Could you check a few things on this model? Use its own coordinates, in mm. Face numbers are marked on the shaded views. A direction names the side the tool comes from. Give positions to 0.01 mm unless a question says otherwise; leave off trailing zeros. Loops run counter-clockwise (first coordinate to the right, second up) from the corner with the lowest first, then second, coordinate; pieces in that order, holes last. Notation, with made-up numbers: (-3.75, 20.25) -> (28.25, 20.25) arc R21 cw to (28.25, 49.25) -> close; hole circle Ø9 at (73, 59). An arc over 180 degrees is marked (long way). Put each result on its own line as item: value.
```python
from build123d import *

# Parameters (mm, degrees)
BOSS_EXTRUDE1_DEPTH = 25.4
SKETCH3_R           = 2.159
CUT_EXTRUDE3_DEPTH  = 49.912809743
CUT_EXTRUDE4_DEPTH  = 49.050496574
CHAMFER1_SIZE       = 3.175


with BuildPart() as part:
    # Sketch2 → Boss-Extrude1 (new, symmetric)
    with BuildSketch(Plane.XY):
        Polygon((-14.859, 0), (-14.225031823, 0), (14.859, 0), (14.859, -26.67), (30.861, -26.67), (30.861, -28.194), (13.335, -28.194), (13.335, -1.524), (-13.335, -1.524), (-13.335, -28.194), (-30.861, -28.194), (-30.861, -26.67), (-14.859, -26.67), align=None)
    extrude(amount=BOSS_EXTRUDE1_DEPTH, both=True)

    # Sketch3 → Cut-Extrude3 (cut, through all)
    with BuildSketch(Plane(origin=(0, 0, 0), x_dir=(1, 0, 0), z_dir=(0, 1, 0))):
        with Locations(Location((0, -15.875, 0), (0, 0, 270))):
            Circle(SKETCH3_R)
        with Locations(Location((0, 15.875, 0), (0, 0, 270))):
            Circle(SKETCH3_R)
        with Locations(Location((0, 0, 0), (0, 0, 270))):
            Circle(SKETCH3_R)
    extrude(amount=-CUT_EXTRUDE3_DEPTH, mode=Mode.SUBTRACT)

    # Sketch9 → Cut-Extrude4 (cut, through all)
    with BuildSketch(Plane(origin=(0, -26.67, 0), x_dir=(1, 0, 0), z_dir=(0, 1, 0))):
        with BuildLine():
            Line((26.4668, 19.0373), (26.4668, 12.7127))
            ThreePointArc((26.4668, 12.7127), (22.8981, 9.144), (19.3294, 12.7127))
            Line((19.3294, 12.7127), (19.3294, 19.0373))
            ThreePointArc((19.3294, 19.0373), (22.8981, 22.606), (26.4668, 19.0373))
        make_face()
        with BuildLine():
            Line((-26.4668, 19.0373), (-26.4668, 12.7127))
            ThreePointArc((-26.4668, 12.7127), (-22.8981, 9.144), (-19.3294, 12.7127))
            Line((-19.3294, 12.7127), (-19.3294, 19.0373))
            ThreePointArc((-19.3294, 19.0373), (-22.8981, 22.606), (-26.4668, 19.0373))
        make_face()
        with BuildLine():
            Line((26.4668, -19.0373), (26.4668, -12.7127))
            ThreePointArc((26.4668, -12.7127), (22.8981, -9.144), (19.3294, -12.7127))
            Line((19.3294, -12.7127), (19.3294, -19.0373))
            ThreePointArc((19.3294, -19.0373), (22.8981, -22.606), (26.4668, -19.0373))
        make_face()
        with BuildLine():
            Line((-26.4668, -19.0373), (-26.4668, -12.7127))
            ThreePointArc((-26.4668, -12.7127), (-22.8981, -9.144), (-19.3294, -12.7127))
            Line((-19.3294, -12.7127), (-19.3294, -19.0373))
            ThreePointArc((-19.3294, -19.0373), (-22.8981, -22.606), (-26.4668, -19.0373))
        make_face()
    extrude(amount=-CUT_EXTRUDE4_DEPTH, mode=Mode.SUBTRACT)

    # Chamfer1
    chamfer1_edges = [part.edges().sort_by_distance(p)[0] for p in [
        (-30.861, -27.432, 25.4),
        (30.861, -27.432, -25.4),
        (-30.861, -27.432, -25.4),
        (30.861, -27.432, 25.4),
    ]]
    chamfer(chamfer1_edges, length=CHAMFER1_SIZE)


solid = part.part
```
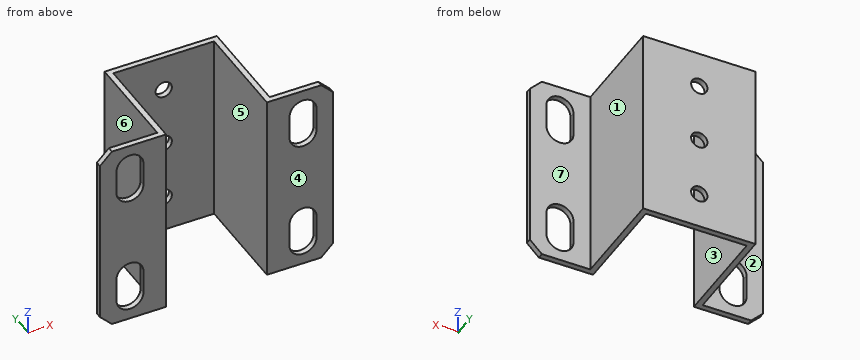
1. Thinking about a two-plate mould opening in X: for the marked faces 1, 2 and 3, which applies, pulls with the +X half, pulls with the -X half, needs draft (parallel to the pull), parting line crosses it, or undercut?
Recorded:
face 1: pulls with the +X half
face 2: needs draft
face 3: undercut
2. If we section it at A-A (y = -21.75): List the corners of the cut face in (x, z) for me (3 decimals), then the cut area to 3 significant figures.
Recorded:
outline: (-14.859, -25.4) -> (-13.335, -25.4) -> (-13.335, 25.4) -> (-14.859, 25.4) -> close; (13.335, -25.4) -> (14.859, -25.4) -> (14.859, 25.4) -> (13.335, 25.4) -> close
area: 155 mm^2
3. If we section it at B-B (x = 0): List the corners of the cut face in (y, z) for me, then the cut area to 3 significant figures.
Recorded:
outline: (-1.52, -25.4) -> (0, -25.4) -> (0, -18.03) -> (-1.52, -18.03) -> close; (-1.52, -13.72) -> (0, -13.72) -> (0, -2.16) -> (-1.52, -2.16) -> close; (-1.52, 2.16) -> (0, 2.16) -> (0, 13.72) -> (-1.52, 13.72) -> close; (-1.52, 18.03) -> (0, 18.03) -> (0, 25.4) -> (-1.52, 25.4) -> close
area: 57.7 mm^2
4. For the marked faces 4, 5, 6 and 7, which set-ups out of +Z, -Z, +X, -X, +Y, -Y let a thin tool reach every point of the face, with its end or its side?
Recorded:
face 4: +Z, -Z, +X, -X, -Y
face 5: +Z, -Z, -Y
face 6: +Z, -Z, -X, +Y
face 7: +Z, -Z, +X, +Y
5. I'm going to push flat-ended pins straight in: pin 1 (8 mm diameter, centred on y = -15, z = -5.5, fed in from +X); pin 2 (8 mm diameter, centred on x = 24.5, z = -2.5, fed in from +Y); pin 3 (3 mm diameter, centred on y = -21.5, z = -15, fed in from -X). Where does each tip first touch, or does it pass through?
Recorded:
pin 1: stops at x = 14.86
pin 2: stops at y = -26.67
pin 3: stops at x = -14.86
6. If we section it at D-D (z = -5.5): List the corners of the cut face in (x, y) for me (3 decimals), then the cut area to 3 significant figures.
Recorded:
outline: (-30.861, -28.194) -> (-13.335, -28.194) -> (-13.335, -1.524) -> (13.335, -1.524) -> (13.335, -28.194) -> (30.861, -28.194) -> (30.861, -26.67) -> (14.859, -26.67) -> (14.859, 0) -> (-14.859, 0) -> (-14.859, -26.67) -> (-30.861, -26.67) -> close
area: 175 mm^2
7. If we section it at C-C (z = 0): List the corners of the cut face in (x, y) for me (3 decimals), then the cut area to 3 significant figures.
Recorded:
outline: (-30.861, -28.194) -> (-13.335, -28.194) -> (-13.335, -1.524) -> (-2.159, -1.524) -> (-2.159, 0) -> (-14.859, 0) -> (-14.859, -26.67) -> (-30.861, -26.67) -> close; (2.159, -1.524) -> (13.335, -1.524) -> (13.335, -28.194) -> (30.861, -28.194) -> (30.861, -26.67) -> (14.859, -26.67) -> (14.859, 0) -> (2.159, 0) -> close
area: 169 mm^2
8. I need wall thicknesses on line 1 (X direction, y = -6.5, z = 16.5) (3 decimals); line 2 (Y direction, x = 19, z = -3); line 3 (Y direction, x = 11.5, z = 9). Which ranges of each line are inside material? Lowest first, please.
Recorded:
line 1: x = -14.859 to -13.335, 13.335 to 14.859
line 2: y = -28.19 to -26.67
line 3: y = -1.52 to 0
